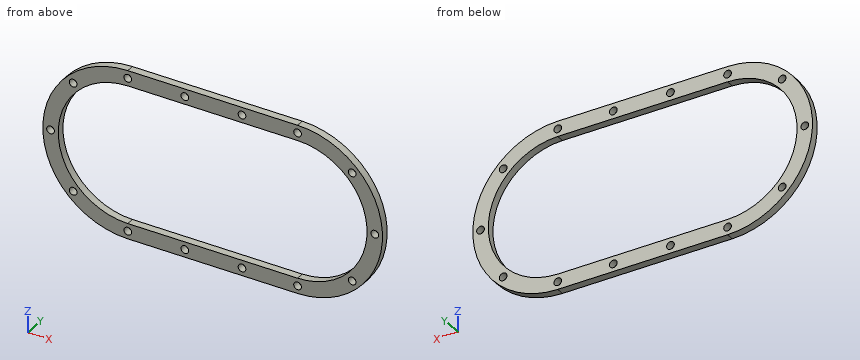
from build123d import *

# Parameters (mm, degrees)
BOSS_EXTRUDE1_DEPTH    = 10
F_10_0MM_DOWEL_HOLE6_D = 10
CIRPATTERN2_COUNT      = 5
CIRPATTERN2_ANGLE      = 180
MIRROR2_COPY_1_D       = 10
MIRROR2_COPY_2_D       = 10
MIRROR2_COPY_3_D       = 10
MIRROR2_COPY_4_D       = 10
LPATTERN1_COUNT        = 3
LPATTERN1_PITCH        = 74
MIRROR3_COPY_1_D       = 10
MIRROR3_COPY_2_D       = 10
MIRROR3_COPY_3_D       = 10


with BuildPart() as part:
    # Sketch1 → Boss-Extrude1 (new body)
    with BuildSketch(Plane(origin=(0, 0, 0), x_dir=(1, 0, 0), z_dir=(0, 1, 0))):
        with BuildLine():
            Line((-110, 110), (110, 110))
            ThreePointArc((110, 110), (220, 0), (110, -110))
            Line((110, -110), (-110, -110))
            ThreePointArc((-110, -110), (-220, 0), (-110, 110))
        make_face()
        with BuildLine():
            Line((-110, 90), (110, 90))
            ThreePointArc((110, 90), (200, 0), (110, -90))
            Line((110, -90), (-110, -90))
            ThreePointArc((-110, -90), (-200, 0), (-110, 90))
        make_face(mode=Mode.SUBTRACT)
    extrude(amount=BOSS_EXTRUDE1_DEPTH)

    # Ø10.0mm Dowel Hole6 (through all)
    with Locations(Plane(origin=(-110, 10, -100), x_dir=(0, 0, 1), z_dir=(0, 1, 0))):
        with Locations((0, 0)):
            f_10_0mm_dowel_hole6 = Hole(F_10_0MM_DOWEL_HOLE6_D / 2)

    # CirPattern2: Ø10.0mm Dowel Hole6 ×5 about axis
    cirpattern2_axis = Axis((-110, 0, 0), (0, 1, 0))
    for i in range(1, CIRPATTERN2_COUNT):
        add(f_10_0mm_dowel_hole6.rotate(cirpattern2_axis, i * CIRPATTERN2_ANGLE / (CIRPATTERN2_COUNT - 1)), mode=Mode.SUBTRACT)

    # Mirror2: Ø10.0mm Dowel Hole6 across plane
    add(f_10_0mm_dowel_hole6.mirror(Plane(origin=(0, 0, 0), x_dir=(0, 0, 1), z_dir=(1, 0, 0))), mode=Mode.SUBTRACT)

    # Mirror2 copy 1 (through all)
    with Locations(Plane(origin=(180.710678119, 10, -70.710678119), x_dir=(-0.707106781, 0, 0.707106781), z_dir=(0, 1, 0))):
        with Locations((0, 0)):
            Hole(MIRROR2_COPY_1_D / 2)

    # Mirror2 copy 2 (through all)
    with Locations(Plane(origin=(210, 10, 0), x_dir=(-1, 0, 0), z_dir=(0, 1, 0))):
        with Locations((0, 0)):
            Hole(MIRROR2_COPY_2_D / 2)

    # Mirror2 copy 3 (through all)
    with Locations(Plane(origin=(180.710678119, 10, 70.710678119), x_dir=(-0.707106781, 0, -0.707106781), z_dir=(0, 1, 0))):
        with Locations((0, 0)):
            Hole(MIRROR2_COPY_3_D / 2)

    # Mirror2 copy 4 (through all)
    with Locations(Plane(origin=(110, 10, 100), x_dir=(0, 0, -1), z_dir=(0, 1, 0))):
        with Locations((0, 0)):
            Hole(MIRROR2_COPY_4_D / 2)

    # LPattern1: Ø10.0mm Dowel Hole6 ×3
    with Locations(*[(i * LPATTERN1_PITCH, 0, 0) for i in range(1, LPATTERN1_COUNT)]):
        add(f_10_0mm_dowel_hole6, mode=Mode.SUBTRACT)

    # Mirror3 copy 1 (through all)
    with Locations(Plane(origin=(-36, 10, 100), x_dir=(0, 0, -1), z_dir=(0, 1, 0))):
        with Locations((0, 0)):
            Hole(MIRROR3_COPY_1_D / 2)

    # Mirror3 copy 2 (through all)
    with Locations(Plane(origin=(38, 10, 100), x_dir=(0, 0, -1), z_dir=(0, 1, 0))):
        with Locations((0, 0)):
            Hole(MIRROR3_COPY_2_D / 2)

    # Mirror3 copy 3 (through all)
    with Locations(Plane(origin=(-110, 10, 100), x_dir=(0, 0, -1), z_dir=(0, 1, 0))):
        with Locations((0, 0)):
            Hole(MIRROR3_COPY_3_D / 2)


solid = part.part
Could you check a few things on this model? Use its own coordinates, in mm. Round coordinates to 2 decimals unless told otherwise and drop trailing zeros. Order: outer loops, then holes, each group sorted by start corner. A loop starts at its lowest first (then second) coordinate and runs counter-clockwise, first axis right, second up.
Q1. Please list where these lines run through material, in increasing order: probe 1 along X at (y, z) = (8.25, -100); probe 2 along Z at (x, y) = (-94, 7.25); probe 3 along Z at (x, y) = (-33, 9.25).
Geometry says:
probe 1: x = -155.83 to -115, -105 to -41, -31 to 33, 43 to 105, 115 to 155.83
probe 2: z = -110 to -90, 90 to 110
probe 3: z = -110 to -104, -96 to -90, 90 to 96, 104 to 110
Q2. Imagine slicing it at B-B, the plane z = -86. List the corners of the cut face in (x, y) for me.
Geometry says:
outline: (-178.59, 0) - (-136.53, 0) - (-136.53, 10) - (-178.59, 10) - close; (136.53, 0) - (178.59, 0) - (178.59, 10) - (136.53, 10) - close
Q3. Imagine slicing it at D-D, the plane y = 6.25. State how many separate pieces and enclosed holes the cut face has, then the cut area to 3 significant figures.
Geometry says:
separate pieces: 1
enclosed holes: 15
area: 20,300 mm2
Q4. I'm going to push flat-ended pins straight in: P1, Ø6, axis at x = -180.71, z = 70.71, coming from the -Y side; P2, Ø1, axis at x = 135.5, y = 2, coming from the +Z side; P3, Ø11.5, axis at x = -210, z = 0, coming from the +Y side; P4, Ø4, axis at y = 3, z = 47.5, coming from the -X side. Where does each tip first touch, or does it pass through?
Geometry says:
P1: passes through
P2: stops at z = 107.12
P3: stops at y = 10
P4: stops at x = -210.15
Q5. Imagine slicing it at C-C, the plane z = 100. List the corners of the cut face in (x, y) for me, then the cut area to 3 significant figures.
Geometry says:
outline: (-155.83, 0) - (-115, 0) - (-115, 10) - (-155.83, 10) - close; (-105, 0) - (-41, 0) - (-41, 10) - (-105, 10) - close; (-31, 0) - (33, 0) - (33, 10) - (-31, 10) - close; (43, 0) - (105, 0) - (105, 10) - (43, 10) - close; (115, 0) - (155.83, 0) - (155.83, 10) - (115, 10) - close
area: 2,720 mm2
Q6. Imagine slicing it at A-A, the plane x = 89. List the corners of the cut face in (y, z) for me.
Geometry says:
outline: (0, -110) - (10, -110) - (10, -90) - (0, -90) - close; (0, 90) - (10, 90) - (10, 110) - (0, 110) - close
